from build123d import *

# Parameters (mm, degrees)
F0_W     = 30
F0_H     = 10
F1_DEPTH = 20
F2_T     = -1.5
F3_R     = 4.99999


# Not quite as in the source:
# - a fillet or chamfer is up to 0.001 mm smaller than in the source, because OpenCascade refuses the exact size


with BuildPart() as f1:
    # F0 (on Top) → F1 (new body)
    with BuildSketch(Plane.XY):
        Rectangle(F0_W, F0_H)
    extrude(amount=F1_DEPTH)

    # F2
    f2_openings = [f1.faces().sort_by_distance(p)[0] for p in [
        (0, 0, 0),
    ]]
    offset(amount=F2_T, openings=f2_openings)

    # F3 (radius 5 in the source; OpenCascade refuses exactly that, so slightly less here)
    f3_edges = [f1.edges().sort_by_distance(p)[0] for p in [
        (-15, 0, 20),
        (0, -5, 20),
        (0, 5, 20),
        (15, 0, 20),
    ]]
    fillet(f3_edges, radius=F3_R)


solid = f1.part
Source: CAD feature listing. Evaluate the final solid. Frame: model axes, mm. A direction names the side the tool comes from. Coordinates: 2 decimals unless noted, no trailing zeros. Loops run counter-clockwise (first coordinate to the right, second up) from the corner with the lowest first, then second, coordinate; pieces in that order, holes last. Notation, with made-up numbers: (69.5, 87) - (125.5, 87) arc R19 cw to (125.5, 120) - close; hole circle Ø10 at (30, 14.5). An arc over 180 degrees is marked (long way). One line per question, with ' | ' between items.
1) Section D-D, the plane z = 17.75. Return loops of the section in (x, y).
Report:
outline: (-14.18, -4.18) - (14.18, -4.18) - (14.18, 4.18) - (-14.18, 4.18) - close; hole (-13.5, -3.5) - (13.5, -3.5) - (13.5, 3.5) - (-13.5, 3.5) - close
2) Pull-direction query (X, two-part tool) for faces 3 (the face through (0, 4, 18)), 4 (the face through (0, -3.5, 9)), 5 (the face through (-15, 0, 7)), 6 (the face through (0, 3.5, 9)); classes: released by +X, released by -X, zero draft, split by the parting line, or undercut.
Report:
face 3: zero draft | face 4: undercut | face 5: released by -X | face 6: undercut
3) Section B-B, the plane z = 3.5. Return loops of the section in (x, y), then the cut area to 3 significant figures.
Report:
outline: (-15, -5) - (15, -5) - (15, 5) - (-15, 5) - close; hole (-13.5, -3.5) - (13.5, -3.5) - (13.5, 3.5) - (-13.5, 3.5) - close | area: 111 mm²
4) First-contact query: P1, Ø2, axis at x = 5.5, y = 0, coming from the -Z side. Flat tip, straight axial feed; report the tip coordinate or a pass-through.
Report:
P1: stops at z = 18.5
5) Section C-C, the plane y = 1.75. Return loops of the section in (x, z).
Report:
outline: (-15, 0) - (-13.5, 0) - (-13.5, 18.5) - (13.5, 18.5) - (13.5, 0) - (15, 0) - (15, 15) arc R5 ccw to (11.75, 19.68) - (-11.75, 19.68) arc R5 ccw to (-15, 15) - close
6) Set-up query: faces 1 (the face through (0, 5, 7)), 2 (the face through (-13.5, 0, 9)). Return all of +Z, -Z, +X, -X, +Y, -Y with unobstructed straight access to the full face (end or side cutting, diameter ignored); none if empty.
Report:
face 1: +Z, -Z, +X, -X, +Y | face 2: -Z
7) Line query: line 1 along X through (y, z) = (1.5, 6.75); line 2 along Y through (x, z) = (-10.25, 10.75); line 3 along X through (y, z) = (-0.75, 16.5). Output: solid intervals per line, ascending.
Report:
line 1: x = -15 to -13.5, 13.5 to 15 | line 2: y = -5 to -3.5, 3.5 to 5 | line 3: x = -14.77 to -13.5, 13.5 to 14.77
